from build123d import *

# Parameters (mm, degrees)
BOSS_EXTRUDE1_DEPTH = 12.7
SKETCH2_R           = 1.85
CUT_EXTRUDE1_DEPTH  = 30.7
SKETCH3_R           = 5.65
CUT_EXTRUDE2_DEPTH  = 15
SKETCH4_R           = 1.55
CUT_EXTRUDE3_DEPTH  = 3
FILLET1_R           = 1


with BuildPart() as part:
    # Sketch1 → Boss-Extrude1 (new body, symmetric)
    with BuildSketch(Plane(origin=(0, 0, 0), x_dir=(1, 0, 0), z_dir=(0, 1, 0))):
        Polygon((-14.85, 0), (14.85, 0), (14.85, -14), (12.85, -14), (12.85, -2), (-12.85, -2), (-12.85, -14), (-14.85, -14), align=None)
    extrude(amount=BOSS_EXTRUDE1_DEPTH, both=True)

    # Sketch2 → Cut-Extrude1 (cut, through all)
    with BuildSketch(Plane.ZY.offset(14.85)):
        with Locations((8, -6)):
            Circle(SKETCH2_R)
        with Locations((8, 6)):
            Circle(SKETCH2_R)
    extrude(amount=-CUT_EXTRUDE1_DEPTH, mode=Mode.SUBTRACT)

    # Sketch3 → Cut-Extrude2 (cut, through all)
    with BuildSketch(Plane(origin=(0, 0, 0), x_dir=(-1, 0, 0), z_dir=(0, 0, -1))):
        Circle(SKETCH3_R)
    extrude(amount=-CUT_EXTRUDE2_DEPTH, mode=Mode.SUBTRACT)

    # Sketch4 → Cut-Extrude3 (cut, through all)
    with BuildSketch(Plane.XY.offset(2)):
        with Locations((-7.78, 7.78)):
            Circle(SKETCH4_R)
        with Locations((-7.78, -7.78)):
            Circle(SKETCH4_R)
        with Locations((7.78, -7.78)):
            Circle(SKETCH4_R)
        with Locations((7.78, 7.78)):
            Circle(SKETCH4_R)
    extrude(amount=-CUT_EXTRUDE3_DEPTH, mode=Mode.SUBTRACT)

    # Fillet1
    fillet1_edges = [part.edges().sort_by_distance(p)[0] for p in [
        (-14.85, 0, 0),
        (14.85, 0, 0),
    ]]
    fillet(fillet1_edges, radius=FILLET1_R)


solid = part.part
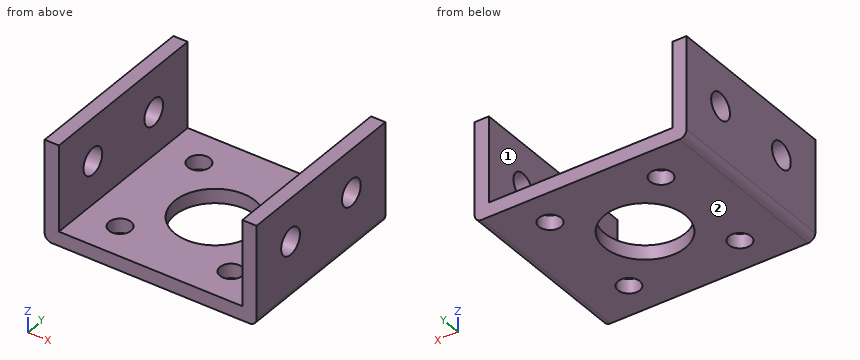
The listing builds one solid part. Answer for the finished solid, in the listing's coordinates (mm). Face numbers are marked on the shaded views. A direction names the side the tool comes from. Round coordinates to 2 decimals unless told otherwise and drop trailing zeros. Loops run counter-clockwise (first coordinate to the right, second up) from the corner with the lowest first, then second, coordinate; pieces in that order, holes last. Notation, with made-up numbers: M 60,-20 L 118,-20 A30 ccw 118,19 Z; hole C -32,59 d11. An arc over 180 degrees is marked long. Return JSON: item names as keys, results as strings.
Q1. This flat-tipped pin is pushed along its axis until it touches: pin 1 Ø3.5 at (x, y) = (7.78, -7.78) entering from +Z. Where does it stop, or does it pass through?
Results list:
{"pin 1": "stops at z = 2"}
Q2. Find section A-A, the plane x = 7.78. Determine the outline of the cut face in (y, z), plus the area to 3 significant figures.
Results list:
{"outline": "M -12.7,0 L -9.33,0 L -9.33,2 L -12.7,2 Z; M -6.23,0 L 6.23,0 L 6.23,2 L -6.23,2 Z; M 9.33,0 L 12.7,0 L 12.7,2 L 9.33,2 Z", "area": "38.4 mm2"}
Q3. Find the intervals of material crossed by line 1 along Y through (x, z) = (7.78, 1.35); line 2 along X through (y, z) = (-3, 13); line 3 along Y through (x, z) = (0, 1), in increasing order. Write a range as from..to.
Results list:
{"line 1": "y = -12.7..-9.33, -6.23..6.23, 9.33..12.7", "line 2": "x = -14.85..-12.85, 12.85..14.85", "line 3": "y = -12.7..-5.65, 5.65..12.7"}
Q4. Which of the six approach directions +Z, -Z, +X, -X, +Y, -Y give full straight-line access (tool end or side, diameter ignored) to the marked faces 1 and 2?
Results list:
{"face 1": "+Z, +Y, -Y", "face 2": "-Z, +X, -X, +Y, -Y"}
Q5. Find section B-B, the plane y = -0.75. Determine the outline of the cut face in (x, z).
Results list:
{"outline": "M -14.85,1 A1 ccw -13.85,0 L -5.6,0 L -5.6,2 L -12.85,2 L -12.85,14 L -14.85,14 Z; M 5.6,0 L 13.85,0 A1 ccw 14.85,1 L 14.85,14 L 12.85,14 L 12.85,2 L 5.6,2 Z"}
Q6. Find section D-D, the plane x = 3.75. Determine the outline of the cut face in (y, z), plus the area to 3 significant figures.
Results list:
{"outline": "M -12.7,0 L -4.23,0 L -4.23,2 L -12.7,2 Z; M 4.23,0 L 12.7,0 L 12.7,2 L 4.23,2 Z", "area": "33.9 mm2"}
Q7. Find section C-C, the plane z = 10.5. Determine the outline of the cut face in (x, y).
Results list:
{"outline": "M -14.85,-12.7 L -12.85,-12.7 L -12.85,12.7 L -14.85,12.7 Z; M 12.85,-12.7 L 14.85,-12.7 L 14.85,12.7 L 12.85,12.7 Z"}
